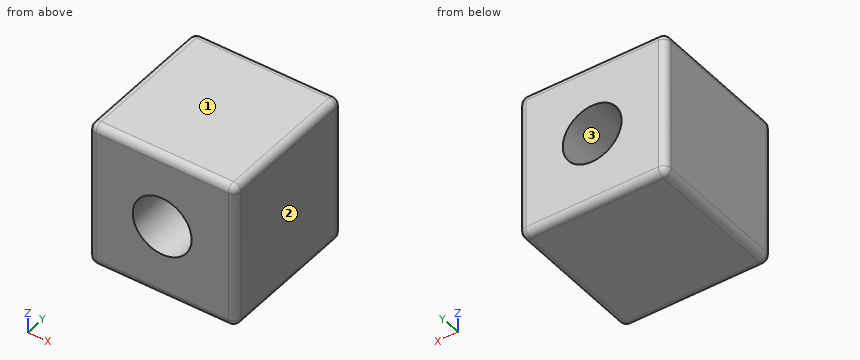
from build123d import *

# Parameters (mm, degrees)
F0_W     = 100
F0_H     = 100
F1_DEPTH = 100
F2_R     = 5
F3_R     = 20
F4_DEPTH = 100


with BuildPart() as f1:
    # F0 (on Front) → F1 (new body)
    with BuildSketch(Plane.XZ):
        with Locations((50, 50)):
            Rectangle(F0_W, F0_H)
    extrude(amount=F1_DEPTH)

    # F2
    f2_edges = [f1.edges().sort_by_distance(p)[0] for p in [
        (50, -100, 100),
        (50, -100, 0),
        (0, -50, 0),
        (0, -100, 50),
        (0, -50, 100),
        (100, -50, 100),
        (50, 0, 100),
        (0, 0, 50),
        (50, 0, 0),
        (100, 0, 50),
        (100, -50, 0),
        (100, -100, 50),
    ]]
    fillet(f2_edges, radius=F2_R)

    # F3 (on face) → F4 (cut)
    with BuildSketch(Plane(origin=(0, 0, 0), x_dir=(-1, 0, 0), z_dir=(0, 1, 0))):
        with Locations((-50, 50)):
            Circle(F3_R)
    extrude(amount=-F4_DEPTH, mode=Mode.SUBTRACT)


solid = f1.part
The listing builds one solid part. Answer for the finished solid, in the listing's coordinates (mm). Face numbers are marked on the shaded views. Round coordinates to 2 decimals unless told otherwise and drop trailing zeros. Order: outer loops, then holes, each group sorted by start corner. A loop starts at its lowest first (then second) coordinate and runs counter-clockwise, first axis right, second up. Notation, with made-up numbers: M 2.25,10 L 10.25,10 A21 cw 10.25,22 Z; hole C -11.5,-2.5 d4. An arc over 180 degrees is marked long. Answer in a Markdown table with one row per item. Add a question column.
1) The part is cut by section C-C on y = -55. Determine the outline of the cut face in (x, z).
2) Consider line 1 along X through (y, z) = (-47.5, 49.5); line 2 along Z through (x, y) = (50, -19.5); line 3 along X through (y, z) = (-27, 63). Determine where each line is inside the solid, lowest interval first. Write a range as from..to.
3) The part is cut by section A-A on x = 50. Determine the outline of the cut face in (y, z).
4) Determine the mould class of the marked faces 1, 2 and 3 for opening direction X: pulls with the +X half, pulls with the -X half, needs draft (parallel to the pull), parting line crosses it, or undercut.
5) The part is cut by section B-B on z = 50. Determine the outline of the cut face in (x, y).
Findings below:
| question | item | result |
|---|---|---|
| 1 | outline | M 0,5 A5 ccw 5,0 L 95,0 A5 ccw 100,5 L 100,95 A5 ccw 95,100 L 5,100 A5 ccw 0,95 Z; hole C 50,50 d40 |
| 2 | line 1 | x = 0..30.01, 69.99..100 |
| 2 | line 2 | z = 0..30, 70..100 |
| 2 | line 3 | x = 0..34.8, 65.2..100 |
| 3 | outline | M -100,5 A5 ccw -95,0 L -5,0 A5 ccw 0,5 L 0,30 L -100,30 Z; M -100,70 L 0,70 L 0,95 A5 ccw -5,100 L -95,100 A5 ccw -100,95 Z |
| 4 | face 1 | needs draft |
| 4 | face 2 | pulls with the +X half |
| 4 | face 3 | undercut |
| 5 | outline | M 0,-95 A5 ccw 5,-100 L 30,-100 L 30,0 L 5,0 A5 ccw 0,-5 Z; M 70,-100 L 95,-100 A5 ccw 100,-95 L 100,-5 A5 ccw 95,0 L 70,0 Z |
